Geometry check sheet. Reference: the model listing, model coordinates, mm. A direction names the side the tool comes from. Give positions to 0.01 mm unless a question says otherwise; leave off trailing zeros. Loops run counter-clockwise (first coordinate to the right, second up) from the corner with the lowest first, then second, coordinate; pieces in that order, holes last. Notation, with made-up numbers: (21, 20) -> (38, 20) arc R35 cw to (38, 53) -> close; hole circle Ø3 at (-27.5, 8.5). An arc over 180 degrees is marked (long way). Answer as a JSON object with one key per item and string values.
from build123d import *

# Parameters (mm, degrees)
F0_W     = 95.3502617776
F0_H     = 133.5505247116
F1_DEPTH = 127
F2_W     = 80.3107917309
F2_H     = 22.5592143834
F2_H_2   = 80.3107880056
F3_DEPTH = 76.2
F4_W     = 80.3107917309
F4_H     = 8.5725001991
F5_DEPTH = 73.66
F6_W     = 86.9281552732
F6_H     = 32.7860526741
F6_W_2   = 80.3107917309
F6_H_2   = 22.5592143834
F7_DEPTH = 127


with BuildPart() as f1:
    # F0 (on Front) → F1 (new body)
    with BuildSketch(Plane.XZ):
        with Locations((-3.3086854964, 0.1503974199)):
            Rectangle(F0_W, F0_H)
    extrude(amount=F1_DEPTH)

    # F2 (on face) → F3 (cut)
    with BuildSketch(Plane.XZ.offset(127)):
        with Locations((-2.1055266261, 48.4271068126)):
            Rectangle(F2_W, F2_H)
        with Locations((-2.1055266261, -17.4457896501)):
            Rectangle(F2_W, F2_H_2)
    extrude(amount=-F3_DEPTH, mode=Mode.SUBTRACT)

    # F4 (on face) → F5 (join)
    with BuildSketch(Plane.XZ.offset(50.8)):
        with Locations((-2.1055266261, -13.1595395505)):
            Rectangle(F4_W, F4_H)
    extrude(amount=F5_DEPTH)

    # F6 (on face) → F7 (join)
    with BuildSketch(Plane.XZ.offset(127)):
        with Locations((-1.8047373742, 47.5247371942)):
            Rectangle(F6_W, F6_H)
        with Locations((-2.1055266261, 48.4271068126)):
            Rectangle(F6_W_2, F6_H_2, mode=Mode.SUBTRACT)
    extrude(amount=F7_DEPTH)


solid = f1.part
1) Depth check by flat-ended pin: P1, Ø1, axis at x = 33.5, z = 47, coming from the +Y side; P2, Ø2, axis at x = -27.5, z = 12, coming from the -Y side; P3, Ø4, axis at x = -15.5, y = -162, coming from the +Z side; P4, Ø3, axis at x = 16, y = -192, coming from the -Z side. Enter the tip coordinate at first touch or a pass-through.
Geometry check:
{"P1": "stops at y = 0", "P2": "stops at y = -50.8", "P3": "stops at z = 63.92", "P4": "stops at z = 31.13"}
2) Section check A-A on y = -151.5. Record the cut outline in (x, z).
Geometry check:
{"outline": "(-45.27, 31.13) -> (41.66, 31.13) -> (41.66, 63.92) -> (-45.27, 63.92) -> close; hole (-42.26, 37.15) -> (38.05, 37.15) -> (38.05, 59.71) -> (-42.26, 59.71) -> close"}
3) Tool access check on faces 4 (the face through (-45.269, -190, 47)), 5 (the face through (-3, -87, -17.446)), 6 (the face through (-2, -190, 31.132)). Record the directions out of +Z, -Z, +X, -X, +Y, -Y that give a thin tool (end or side, any length) a straight path to the whole face; none if there is none.
Geometry check:
{"face 4": "+Z, -Z, -X, -Y", "face 5": "-Y", "face 6": "-Z, +X, -X, -Y"}
4) Material ranges on line 1 along Z through (x, y) = (-0.5, -112.5); line 2 along Z through (x, y) = (-7.5, -163); line 3 along X through (y, z) = (-95.5, -28), recorded low to high. Write a range as from..to.
Geometry check:
{"line 1": "z = -66.62..-57.6, -17.45..-8.87, 22.71..37.15, 59.71..66.93", "line 2": "z = 31.13..37.15, 59.71..63.92", "line 3": "x = -50.98..-42.26, 38.05..44.37"}
5) Section check B-B on z = -47. Record the cut outline in (x, y).
Geometry check:
{"outline": "(-50.98, -127) -> (-42.26, -127) -> (-42.26, -50.8) -> (38.05, -50.8) -> (38.05, -127) -> (44.37, -127) -> (44.37, 0) -> (-50.98, 0) -> close"}
6) Draft check along X on faces 1 (the face through (-3, -50.8, 7)), 2 (the face through (41.659, -190, 47)), 3 (the face through (-8.4, -254, 36.7)). Enter one of: pulls with the +X half, pulls with the -X half, needs draft (parallel to the pull), parting line crosses it, or undercut.
Geometry check:
{"face 1": "undercut", "face 2": "pulls with the +X half", "face 3": "needs draft"}
7) Section check C-C on y = -76.5. Record the cut outline in (x, z).
Geometry check:
{"outline": "(-50.98, -66.62) -> (44.37, -66.62) -> (44.37, 66.93) -> (-50.98, 66.93) -> close; hole (-42.26, -57.6) -> (38.05, -57.6) -> (38.05, -17.45) -> (-42.26, -17.45) -> close; hole (-42.26, -8.87) -> (38.05, -8.87) -> (38.05, 22.71) -> (-42.26, 22.71) -> close; hole (-42.26, 37.15) -> (38.05, 37.15) -> (38.05, 59.71) -> (-42.26, 59.71) -> close"}
8) Section check D-D on x = 9. Record the cut outline in (y, z), plus the area to 3 significant figures.
Geometry check:
{"outline": "(-254, 31.13) -> (-127, 31.13) -> (-127, 22.71) -> (-50.8, 22.71) -> (-50.8, -8.87) -> (-124.46, -8.87) -> (-124.46, -17.45) -> (-50.8, -17.45) -> (-50.8, -57.6) -> (-127, -57.6) -> (-127, -66.62) -> (0, -66.62) -> (0, 66.93) -> (-127, 66.93) -> (-127, 63.92) -> (-254, 63.92) -> (-254, 59.71) -> (-50.8, 59.71) -> (-50.8, 37.15) -> (-254, 37.15) -> close", "area": "11,100 mm2"}
